from build123d import *

# Parameters (mm, degrees)
CYLINDER001_R     = 1.7
CYLINDER001_DEPTH = 31
CYLINDER_R        = 1.7
CYLINDER_DEPTH    = 31
BOX003_W          = 3
BOX003_H          = 30
BOX003_DEPTH      = 19
BOX001_W          = 12
BOX001_H          = 27
BOX001_DEPTH      = 3
BOX002_W          = 12
BOX002_H          = 27
BOX002_DEPTH      = 3
BOX_W             = 95
BOX_H             = 3
BOX_DEPTH         = 19
FILLET_R          = 5


with BuildPart() as cylinder001:
    # Cylinder001 → Cylinder001 (new body)
    with BuildSketch(Plane(origin=(6, 23.2, -6), x_dir=(1, 0, 0), z_dir=(0, 0, 1))):
        Circle(CYLINDER001_R)
    extrude(amount=CYLINDER001_DEPTH)


with BuildPart() as obj1:
    # Cylinder → Cylinder (new body)
    with BuildSketch(Plane(origin=(6, 5.5, -6), x_dir=(1, 0, 0), z_dir=(0, 0, 1))):
        Circle(CYLINDER_R)
    extrude(amount=CYLINDER_DEPTH)

    # Fusion001: union Cylinder001
    add(cylinder001.part)


with BuildPart() as cube003:
    # Box003 → Box003 (new body)
    with BuildSketch(Plane(origin=(78, 0, 0), x_dir=(1, 0, 0), z_dir=(0, 0, 1))):
        with Locations((1.5, 15)):
            Rectangle(BOX003_W, BOX003_H)
    extrude(amount=BOX003_DEPTH)


with BuildPart() as cube001:
    # Box001 → Box001 (new body)
    with BuildSketch(Plane.XY.offset(-3)):
        with Locations((6, 13.5)):
            Rectangle(BOX001_W, BOX001_H)
    extrude(amount=BOX001_DEPTH)


with BuildPart() as cube002:
    # Box002 → Box002 (new body)
    with BuildSketch(Plane.XY.offset(19)):
        with Locations((6, 13.5)):
            Rectangle(BOX002_W, BOX002_H)
    extrude(amount=BOX002_DEPTH)


with BuildPart() as cut:
    # Box → Box (new body)
    with BuildSketch(Plane(origin=(-17, 0, 0), x_dir=(1, 0, 0), z_dir=(0, 0, 1))):
        with Locations((47.5, 1.5)):
            Rectangle(BOX_W, BOX_H)
    extrude(amount=BOX_DEPTH)

    # Fusion: union Cube003, Cube001, Cube002
    add(cube003.part)
    add(cube001.part)
    add(cube002.part)

    # Fillet
    fillet_edges = [cut.edges().sort_by_distance(p)[0] for p in [
        (79.5, 30, 0),
        (79.5, 30, 19),
        (0, 27, 20.5),
        (12, 27, 20.5),
        (-17, 1.5, 19),
        (-17, 1.5, 0),
        (0, 27, -1.5),
        (12, 27, -1.5),
    ]]
    fillet(fillet_edges, radius=FILLET_R)

    # Cut: cut obj1
    add(obj1.part, mode=Mode.SUBTRACT)


solid = cut.part
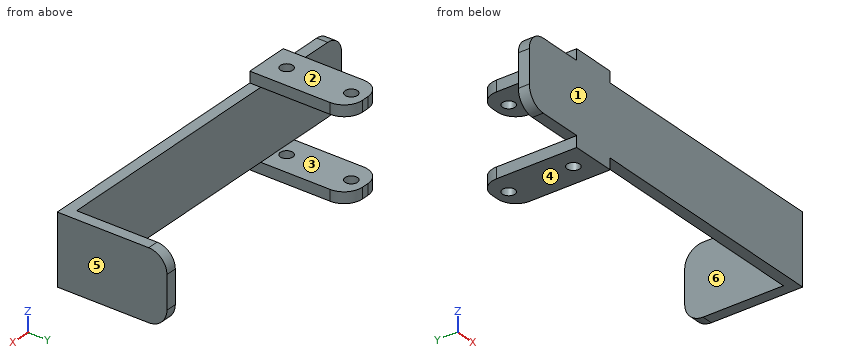
CAD build for the part. Positions are in the model's coordinates, mm. Face numbers are marked on the shaded views. A direction names the side the tool comes from. Give positions to 0.01 mm unless a question says otherwise; leave off trailing zeros. Write each loop counter-clockwise with the first axis right and the second up, starting at its lowest first coordinate (ties: lowest second). Pieces come first, ordered by that corner, then holes. Notation, with made-up numbers: (-20, -3) - (-2, -3) arc R35 ccw to (-2, 31) - close; hole circle Ø2 at (32.25, 56.25). An arc over 180 degrees is marked (long way). Put each result on its own line as item: value.
(1) Saw through at A-A (y = 5.5). List the corners of the cut face in (x, z).
Working result:
outline: (0, -3) - (4.3, -3) - (4.3, 0) - (0, 0) - close; (0, 19) - (4.3, 19) - (4.3, 22) - (0, 22) - close; (7.7, -3) - (12, -3) - (12, 0) - (7.7, 0) - close; (7.7, 19) - (12, 19) - (12, 22) - (7.7, 22) - close; (78, 0) - (81, 0) - (81, 19) - (78, 19) - close
(2) Saw through at B-B (x = 6). List the corners of the cut face in (y, z), then the cut area to 3 significant figures.
Working result:
outline: (0, -3) - (3.8, -3) - (3.8, 0) - (3, 0) - (3, 19) - (3.8, 19) - (3.8, 22) - (0, 22) - close; (7.2, -3) - (21.5, -3) - (21.5, 0) - (7.2, 0) - close; (7.2, 19) - (21.5, 19) - (21.5, 22) - (7.2, 22) - close; (24.9, -3) - (27, -3) - (27, 0) - (24.9, 0) - close; (24.9, 19) - (27, 19) - (27, 22) - (24.9, 22) - close
area: 178 mm^2
(3) Drop flat-ended pins along their axis: pin 1 Ø5.5 at (x, y) = (6, 5.5) entering from -Z; pin 2 Ø0.9 at (y, z) = (13.5, 20) entering from +X; pin 3 Ø2.5 at (x, y) = (6, 23.2) entering from -Z; pin 4 Ø3 at (x, z) = (-1, 5) entering from +Y. Give the stop position or say it passes through.
Working result:
pin 1: z = -3
pin 2: x = 12
pin 3: through
pin 4: y = 3
(4) Wall check: L1, parallel to Y at x = 6, z = -1; L2, parallel to X at y = 5.5, z = 21.25; L3, parallel to Y at x = 42, z = 12. Give the ranges that are in metal, low to high.
Working result:
L1: 0 to 3.8, 7.2 to 21.5, 24.9 to 27
L2: 0 to 4.3, 7.7 to 12
L3: 0 to 3
(5) Saw through at C-C (y = 19.25). List the corners of the cut face in (x, z), then the cut area to 3 significant figures.
Working result:
outline: (0, -3) - (12, -3) - (12, 0) - (0, 0) - close; (0, 19) - (12, 19) - (12, 22) - (0, 22) - close; (78, 0) - (81, 0) - (81, 19) - (78, 19) - close
area: 129 mm^2
(6) Tool access for the marked faces 5 and 6: list every direction of +Z, -Z, +X, -X, +Y, -Y with a clear straight run to the whole face (end or side of a thin tool).
Working result:
face 5: +Z, -Z, +X, +Y, -Y
face 6: +Z, -Z, -X, +Y
(7) Saw through at D-D (z = 20.25). List the corners of the cut face in (x, y).
Working result:
outline: (0, 0) - (12, 0) - (12, 22) arc R5 ccw to (7, 27) - (5, 27) arc R5 ccw to (0, 22) - close; hole circle Ø3.4 at (6, 5.5); hole circle Ø3.4 at (6, 23.2)
(8) Pull direction Z, two halves, no side cores. Call the marked faces 1, 2, 3 and 4: released by +Z, released by -Z, zero draft, split by the parting line, or undercut.
Working result:
face 1: zero draft
face 2: released by +Z
face 3: undercut
face 4: released by -Z
